Here's how the part is built. I have some questions about the finished solid (model axes, mm). Face numbers are marked on the shaded views. A direction names the side the tool comes from. Give positions to 0.01 mm unless a question says otherwise; leave off trailing zeros. Loops run counter-clockwise (first coordinate to the right, second up) from the corner with the lowest first, then second, coordinate; pieces in that order, holes last.
Q1. If we section it at A-A (x = 51): Please give me the cut outline in (y, z).
Q2. For the marked faces 4 and 5, which set-ups out of +Z, -Z, +X, -X, +Y, -Y let a thin tool reach every point of the face, with its end or its side?
Q3. I need wall thicknesses on line 1 (X direction, y = -1, z = 32); line 2 (Z direction, x = 38, y = -12.5); line 3 (X direction, y = -1, z = 83). Which ranges of each line are inside material? Lowest first, please.
Q4. If we section it at B-B (z = 11): Give the number of separate pieces and of enclosed holes in the cut face, plus the area to 3 significant figures.
Q5. We'd pull the mould along X, two halves only. Please class the marked faces 1, 2 and 3: +X half, -X half, draft (parallel to the pull), parting line (faces both ways), or undercut.
Q6. Will these pins go through, and if not, where does the flat tip stop? P1, Ø6, axis at x = 6.5, z = 107, coming from the -Y side; P2, Ø8, axis at x = -8.5, z = 98, coming from the +Y side; P3, Ø4.5, axis at x = 0, z = 115, coming from the +Y side; P4, Ø4, axis at x = 40, y = 14.5, coming from the +Z side.
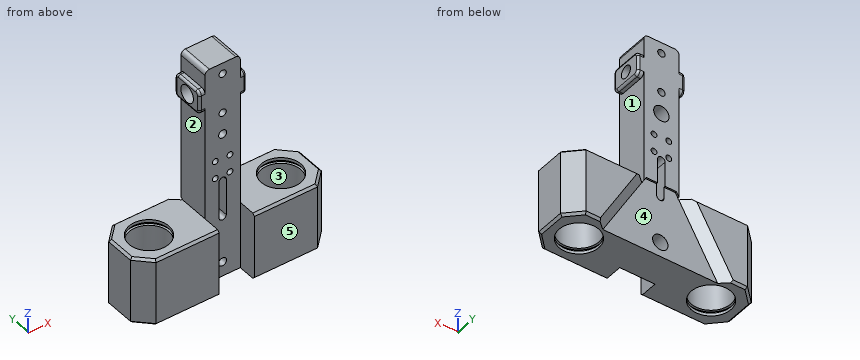
from build123d import *

# Parameters (mm, degrees)
SKETCH1_W           = 130
SKETCH1_H           = 40
BOSS_EXTRUDE1_DEPTH = 125
SKETCH2_R           = 13.5
CUT_EXTRUDE1_DEPTH  = 130
SKETCH3_W           = 24
SKETCH3_H           = 13
CUT_EXTRUDE2_DEPTH  = 125
SKETCH4_W           = 20.5
SKETCH4_H           = 5
CUT_EXTRUDE3_DEPTH  = 125
SKETCH5_R           = 2.75
CUT_EXTRUDE4_DEPTH  = 40
SKETCH6_R           = 2
CUT_EXTRUDE5_DEPTH  = 40
SKETCH7_R           = 5.25
CUT_EXTRUDE6_DEPTH  = 15
CUT_EXTRUDE11_START = -4
SKETCH10_R          = 15
SKETCH10_R_2        = 13.5
CUT_EXTRUDE11_DEPTH = 2
CHAMFER1_SIZE       = 10
CUT_EXTRUDE13_DEPTH = 79
CUT_EXTRUDE14_START = -2
SKETCH13_R          = 15
SKETCH13_R_2        = 13.5
CUT_EXTRUDE14_DEPTH = 2
CUT_EXTRUDE16_DEPTH = 6
CHAMFER2_SIZE       = 6
CHAMFER3_SIZE       = 1.5
CHAMFER4_SIZE       = 1.5
SKETCH16_W          = 24
SKETCH16_H          = 22
BOSS_EXTRUDE2_DEPTH = 25
SKETCH17_R          = 2.5
CUT_EXTRUDE17_DEPTH = 25
FILLET2_R           = 3
SKETCH18_W          = 32
SKETCH18_H          = 16
BOSS_EXTRUDE3_DEPTH = 22
SKETCH19_R          = 4.2
CUT_EXTRUDE18_DEPTH = 40
FILLET3_R           = 3
FILLET4_R           = 1.5
SKETCH20_R          = 5.75
CUT_EXTRUDE19_DEPTH = 11


with BuildPart() as part:
    # Sketch1 → Boss-Extrude1 (new body)
    with BuildSketch(Plane.XY):
        Rectangle(SKETCH1_W, SKETCH1_H)
    extrude(amount=BOSS_EXTRUDE1_DEPTH)

    # Sketch2 → Cut-Extrude1 (cut)
    with BuildSketch(Plane.XY.offset(125)):
        with Locations((-45, 0)):
            Circle(SKETCH2_R)
        with Locations((45, 0)):
            Circle(SKETCH2_R)
    extrude(amount=-CUT_EXTRUDE1_DEPTH, mode=Mode.SUBTRACT)

    # Sketch3 → Cut-Extrude2 (cut)
    with BuildSketch(Plane.XY.offset(125)):
        with Locations((0, -13.5)):
            Rectangle(SKETCH3_W, SKETCH3_H)
    extrude(amount=-CUT_EXTRUDE2_DEPTH, mode=Mode.SUBTRACT)

    # Sketch4 → Cut-Extrude3 (cut)
    with BuildSketch(Plane.XY.offset(125)):
        with Locations((0, 17.5)):
            Rectangle(SKETCH4_W, SKETCH4_H)
    extrude(amount=-CUT_EXTRUDE3_DEPTH, mode=Mode.SUBTRACT)

    # Sketch5 → Cut-Extrude4 (cut)
    with BuildSketch(Plane(origin=(0, 15, 0), x_dir=(1, 0, 0), z_dir=(0, 1, 0))):
        with Locations(Location((0, -10, 0), (0, 0, 270))):
            Circle(SKETCH5_R)
        with Locations(Location((0, -100, 0), (0, 0, 270))):
            Circle(SKETCH5_R)
    extrude(amount=-CUT_EXTRUDE4_DEPTH, mode=Mode.SUBTRACT)

    # Sketch6 → Cut-Extrude5 (cut)
    with BuildSketch(Plane(origin=(0, 15, 0), x_dir=(1, 0, 0), z_dir=(0, 1, 0))):
        with Locations(Location((-5, -71, 0), (0, 0, 270))):
            Circle(SKETCH6_R)
        with Locations(Location((5, -71, 0), (0, 0, 270))):
            Circle(SKETCH6_R)
        with Locations(Location((5, -83, 0), (0, 0, 270))):
            Circle(SKETCH6_R)
        with Locations(Location((-5, -83, 0), (0, 0, 270))):
            Circle(SKETCH6_R)
        with BuildLine():
            Line((2.5, -42), (2.5, -67))
            ThreePointArc((2.5, -67), (0, -69.5), (-2.5, -67))
            Line((-2.5, -67), (-2.5, -42))
            ThreePointArc((-2.5, -42), (0, -39.5), (2.5, -42))
        make_face()
    extrude(amount=-CUT_EXTRUDE5_DEPTH, mode=Mode.SUBTRACT)

    # Sketch7 → Cut-Extrude6 (cut)
    with BuildSketch(Plane(origin=(0, 15, 0), x_dir=(1, 0, 0), z_dir=(0, 1, 0))):
        with Locations(Location((0, -100, 0), (0, 0, 270))):
            Circle(SKETCH7_R)
        with Locations(Location((0, -10, 0), (0, 0, 270))):
            Circle(SKETCH7_R)
    extrude(amount=-CUT_EXTRUDE6_DEPTH, mode=Mode.SUBTRACT)

    # Sketch10 → Cut-Extrude11 (cut)
    # profile 1 of 2: a face of its own
    with BuildSketch(Plane(origin=(0, 0, 0), x_dir=(-1, 0, 0), z_dir=(0, 0, -1)).offset(CUT_EXTRUDE11_START)):
        with Locations((-45, 0)):
            Circle(SKETCH10_R)
        with Locations(Location((-45, 0, 0), (0, 0, 180))):
            Circle(SKETCH10_R_2, mode=Mode.SUBTRACT)
    # profile 2 of 2: a face of its own
    with BuildSketch(Plane(origin=(0, 0, 0), x_dir=(-1, 0, 0), z_dir=(0, 0, -1)).offset(CUT_EXTRUDE11_START)):
        with Locations((45, 0)):
            Circle(SKETCH10_R)
        with Locations(Location((45, 0, 0), (0, 0, 180))):
            Circle(SKETCH10_R_2, mode=Mode.SUBTRACT)
    extrude(amount=CUT_EXTRUDE11_DEPTH, mode=Mode.SUBTRACT)

    # Chamfer1
    chamfer1_edges = [part.edges().sort_by_distance(p)[0] for p in [
        (65, -20, 62.5),
        (-65, -20, 62.5),
        (-65, 20, 62.5),
        (65, 20, 62.5),
    ]]
    chamfer(chamfer1_edges, length=CHAMFER1_SIZE)

    # Sketch12 → Cut-Extrude13 (cut)
    with BuildSketch(Plane.XY.offset(125)):
        Polygon((-12, -7), (-12, 15), (-10.25, 15), (-10.25, 20), (-55, 20), (-65, 10), (-65, -10), (-55, -20), (-12, -20), align=None)
        Polygon((12, -7), (12, 15), (10.25, 15), (10.25, 20), (55, 20), (65, 10), (65, -10), (55, -20), (12, -20), align=None)
    extrude(amount=-CUT_EXTRUDE13_DEPTH, mode=Mode.SUBTRACT)

    # Sketch13 → Cut-Extrude14 (cut)
    # profile 1 of 2: a face of its own
    with BuildSketch(Plane.XY.offset(46).offset(CUT_EXTRUDE14_START)):
        with Locations(Location((-45, 0, 0), (0, 0, 180))):
            Circle(SKETCH13_R)
        with Locations((-45, 0)):
            Circle(SKETCH13_R_2, mode=Mode.SUBTRACT)
    # profile 2 of 2: a face of its own
    with BuildSketch(Plane.XY.offset(46).offset(CUT_EXTRUDE14_START)):
        with Locations(Location((45, 0, 0), (0, 0, 180))):
            Circle(SKETCH13_R)
        with Locations((45, 0)):
            Circle(SKETCH13_R_2, mode=Mode.SUBTRACT)
    extrude(amount=-CUT_EXTRUDE14_DEPTH, mode=Mode.SUBTRACT)

    # Sketch14 → Cut-Extrude16 (cut)
    with BuildSketch(Plane(origin=(0, 20, 0), x_dir=(1, 0, 0), z_dir=(0, 1, 0))):
        Polygon((-10.25, -50), (10.25, -50), (39.117513459, 0), (10.25, 0), (-10.25, 0), (-39.117513459, 0), align=None)
    extrude(amount=-CUT_EXTRUDE16_DEPTH, mode=Mode.SUBTRACT)

    # Chamfer2
    chamfer2_edges = [part.edges().sort_by_distance(p)[0] for p in [
        (-25.838457268, 20, 23),
        (25.838457268, 20, 23),
    ]]
    chamfer(chamfer2_edges, length=CHAMFER2_SIZE - 0.0001)  # a hair under: the kernel refuses the full size

    # Chamfer3
    chamfer3_edges = [part.edges().sort_by_distance(p)[0] for p in [
        (-33.5, -20, 46),
        (-60, -15, 46),
        (-65, 0, 46),
        (-60, 15, 46),
        (37.243744418, 20, 46),
        (60, 15, 46),
        (65, 0, 46),
        (60, -15, 46),
        (33.5, -20, 46),
        (-37.243744418, 20, 46),
    ]]
    chamfer(chamfer3_edges, length=CHAMFER3_SIZE)

    # Chamfer4
    chamfer4_edges = [part.edges().sort_by_distance(p)[0] for p in [
        (65, 0, 0),
        (50.52280061, 20, 0),
        (-33.5, -20, 0),
        (-65, 0, 0),
        (-60, 15, 0),
        (-60, -15, 0),
        (60, 15, 0),
        (60, -15, 0),
        (33.5, -20, 0),
        (-50.52280061, 20, 0),
    ]]
    chamfer(chamfer4_edges, length=CHAMFER4_SIZE)

    # Sketch16 → Boss-Extrude2 (add)
    with BuildSketch(Plane.XY.offset(125)):
        with Locations((0, 4)):
            Rectangle(SKETCH16_W, SKETCH16_H)
    extrude(amount=BOSS_EXTRUDE2_DEPTH)

    # Sketch17 → Cut-Extrude17 (cut)
    with BuildSketch(Plane(origin=(0, 15, 0), x_dir=(1, 0, 0), z_dir=(0, 1, 0))):
        with Locations(Location((0, -142.5, 0), (0, 0, 270))):
            Circle(SKETCH17_R)
        with Locations(Location((0, -115, 0), (0, 0, 270))):
            Circle(SKETCH17_R)
    extrude(amount=-CUT_EXTRUDE17_DEPTH, mode=Mode.SUBTRACT)

    # Fillet2
    fillet2_edges = [part.edges().sort_by_distance(p)[0] for p in [
        (12, 4, 150),
        (-12, 4, 150),
    ]]
    fillet(fillet2_edges, radius=FILLET2_R)

    # Sketch18 → Boss-Extrude3 (add)
    with BuildSketch(Plane(origin=(0, 15, 0), x_dir=(1, 0, 0), z_dir=(0, 1, 0))):
        with Locations((0, -128.75)):
            Rectangle(SKETCH18_W, SKETCH18_H)
    extrude(amount=-BOSS_EXTRUDE3_DEPTH)

    # Sketch19 → Cut-Extrude18 (cut)
    with BuildSketch(Plane.ZY.offset(16)):
        with Locations((128.75, 4)):
            Circle(SKETCH19_R)
    extrude(amount=-CUT_EXTRUDE18_DEPTH, mode=Mode.SUBTRACT)

    # Fillet3
    fillet3_edges = [part.edges().sort_by_distance(p)[0] for p in [
        (-14, -7, 120.75),
        (14, -7, 120.75),
        (-14, -7, 136.75),
        (14, -7, 136.75),
        (-14, 15, 120.75),
        (-14, 15, 136.75),
        (14, 15, 136.75),
        (14, 15, 120.75),
    ]]
    fillet(fillet3_edges, radius=FILLET3_R)

    # Fillet4
    fillet4_edges = [part.edges().sort_by_distance(p)[0] for p in [
        (16, 4, 120.75),
        (-16, -7, 128.75),
        (16, -7, 128.75),
        (16, 15, 128.75),
        (16, 4, 136.75),
        (16, 14.121320344, 121.628679656),
        (16, 14.121320344, 135.871320344),
        (16, -6.121320344, 135.871320344),
        (16, -6.121320344, 121.628679656),
        (-16, 4, 136.75),
        (-16, 15, 128.75),
        (-16, 4, 120.75),
        (-16, 14.121320344, 121.628679656),
        (-16, 14.121320344, 135.871320344),
        (-16, -6.121320344, 121.628679656),
        (-16, -6.121320344, 135.871320344),
    ]]
    fillet(fillet4_edges, radius=FILLET4_R)

    # Sketch20 → Cut-Extrude19 (cut)
    with BuildSketch(Plane.ZY.offset(16)):
        with Locations((128.75, 4)):
            Circle(SKETCH20_R)
    extrude(amount=-CUT_EXTRUDE19_DEPTH, mode=Mode.SUBTRACT)


solid = part.part
Check sheet entries:
1. outline: (-20, 1.5) - (-18.5, 0) - (-12.09, 0) - (-12.09, 2) - (-13.75, 2) - (-13.75, 4) - (-12.09, 4) - (-12.09, 42) - (-13.75, 42) - (-13.75, 44) - (-12.09, 44) - (-12.09, 46) - (-18.5, 46) - (-20, 44.5) - close; (12.09, 0) - (18.5, 0) - (20, 1.5) - (20, 44.5) - (18.5, 46) - (12.09, 46) - (12.09, 44) - (13.75, 44) - (13.75, 42) - (12.09, 42) - (12.09, 4) - (13.75, 4) - (13.75, 2) - (12.09, 2) - close
2. face 4: -Z, +Y
2. face 5: +Z, -Z, +X, -X, -Y
3. line 1: x = -65 to -58.46, -31.54 to 31.54, 58.46 to 65
3. line 2: z = 0 to 2, 4 to 42, 44 to 46
3. line 3: x = -12 to -7, -3 to 3, 7 to 12
4. separate pieces: 2
4. enclosed holes: 2
4. area: 2,930 mm2
5. face 1: +X half
5. face 2: -X half
5. face 3: undercut
6. P1: stops at y = -7
6. P2: stops at y = 15
6. P3: passes through
6. P4: stops at z = 46
